from build123d import *

# Parameters (mm, degrees)
F0_W     = 120
F0_H     = 16
F1_DEPTH = 16
F3_D     = 5
F3_DEPTH = 14
F3_TIP   = 1.5021515476
F4_SIZE  = 0.25


with BuildPart() as f1:
    # F0 (on Front) → F1 (new body)
    with BuildSketch(Plane.XZ):
        with Locations((15.7382229716, -3.3073185302)):
            Rectangle(F0_W, F0_H)
    extrude(amount=F1_DEPTH)

    # F3
    with Locations(Plane.XZ.offset(16)):
        with Locations((-17.2617770284, -3.3073185302), (-36.2617770284, -3.3073185302)):
            Hole(F3_D / 2, depth=F3_DEPTH)
            with Locations((0, 0, -(F3_DEPTH + F3_TIP / 2))):  # 118° drill point
                Cone(0, F3_D / 2, F3_TIP, mode=Mode.SUBTRACT)

    # F4
    f4_edges = [f1.edges().sort_by_distance(p)[0] for p in [
        (75.738223, -8, 4.692681),
        (-44.261777, -8, 4.692681),
        (15.738223, 0, 4.692681),
        (15.738223, -16, 4.692681),
        (75.738223, -16, -3.307319),
        (15.738223, -16, -11.307319),
        (-44.261777, -16, -3.307319),
        (-38.761777, -16, -3.307319),
        (-19.761777, -16, -3.307319),
        (-44.261777, -8, -11.307319),
        (-44.261777, 0, -3.307319),
        (75.738223, 0, -3.307319),
        (15.738223, 0, -11.307319),
        (75.738223, -8, -11.307319),
    ]]
    chamfer(f4_edges, length=F4_SIZE)


solid = f1.part
Build history of the part. All positions in model axes, mm. A direction names the side the tool comes from. Round coordinates to 2 decimals unless told otherwise and drop trailing zeros. Loops run counter-clockwise (first coordinate to the right, second up) from the corner with the lowest first, then second, coordinate; pieces in that order, holes last. Notation, with made-up numbers: (88, -17.75) -> (96, -17.75) arc R19 ccw to (96, 9.25) -> close; hole circle Ø10 at (48.5, 51.5). An arc over 180 degrees is marked (long way). Answer in a Markdown table with one row per item.
Item 1: Drill centre lines: L1, parallel to X at y = -7.75, z = -3.5; L2, parallel to X at y = -2.5, z = -5. Where is each one in solid material? Low to high. Write a range as [from, to].
Answers below:
| item | result |
|---|---|
| L1 | x = [-44.26, -38.75], [-33.77, -19.75], [-14.77, 75.74] |
| L2 | x = [-44.26, -38.1], [-34.42, -19.1], [-15.42, 75.74] |
Item 2: Mould opens along X. For faces 3 (the flat face through (15, -8, -11.307)), 4 (the flat face through (-44.262, -8, -3)), 5 (the cylindrical face through (-33.764, -8.779, -3.197)) say: +X half, -X half, draft (parallel to the pull), parting line (faces both ways), or undercut.
Answers below:
| item | result |
|---|---|
| face 3 | draft |
| face 4 | -X half |
| face 5 | undercut |
Item 3: Pin check, flat tips, straight feed: pin 1 (4.5 mm diameter, centred on x = -36.26, z = -3.31, fed in from -Y); pin 2 (2 mm diameter, centred on x = -18.5, z = -4, fed in from -Y). Stop position of each tip, or through.
Answers below:
| item | result |
|---|---|
| pin 1 | stops at y = -1.85 |
| pin 2 | stops at y = -1.95 |
Item 4: Which spindle directions (+Z, -Z, +X, -X, +Y, -Y) get a long thin tool onto all of the face, cutting with end or side? Do faces 1 (the flat face through (15, 0, -3)), 2 (the cylindrical face through (-18.61, -8.78, -1.2)). Say none if no direction does.
Answers below:
| item | result |
|---|---|
| face 1 | +Z, -Z, +X, -X, +Y |
| face 2 | -Y |
Item 5: Saw through at A-A (y = -7.25). Write the cut outline in (x, z).
Answers below:
| item | result |
|---|---|
| outline | (-44.26, -11.06) -> (-44.01, -11.31) -> (75.49, -11.31) -> (75.74, -11.06) -> (75.74, 4.44) -> (75.49, 4.69) -> (-44.01, 4.69) -> (-44.26, 4.44) -> close; hole circle Ø5 at (-36.26, -3.31); hole circle Ø5 at (-17.26, -3.31) |
